Autodesk Inventor part; units mm, degrees
ref_plane "YZ Plane" through (0, 0, 0) normal (1, 0, 0) x (0, 1, 0)
ref_plane "XZ Plane" through (0, 0, 0) normal (0, 1, 0) x (-1, 0, 0)
ref_plane "XY Plane" through (0, 0, 0) normal (0, 0, 1) x (1, 0, 0)
sketch "Sketch1" plane through (0, 0, 0) normal (1, 0, 0) x (0, 1, 0)
  line L0 (35.589, 28.7672) -> (-47.596, 28.7672)
  line L1 (-47.596, 28.7672) -> (-47.596, 3.3672)
  line L2 (-47.596, 3.3672) -> (35.589, 3.3672)
  line L3 (35.589, 3.3672) -> (35.589, 28.7672)
  line L4 (-47.596, 20.8297) -> (-50.771, 20.8297)
  line L5 (-50.771, 20.8297) -> (-50.771, 11.3047)
  line L6 (-50.771, 11.3047) -> (-47.596, 11.3047)
  line L7 (-47.596, 11.3047) -> (-47.596, 20.8297)
  line L8 (-39.6585, 28.7672) -> (-30.1335, 28.7672)
  line L9 (-30.1335, 28.7672) -> (-30.1335, 25.5922)
  line L10 (-30.1335, 25.5922) -> (-39.6585, 25.5922)
  line L11 (-39.6585, 25.5922) -> (-39.6585, 28.7672)
  line L12 (-22.196, 20.8297) -> (-25.371, 20.8297)
  line L13 (-25.371, 20.8297) -> (-25.371, 11.3047)
  line L14 (-25.371, 11.3047) -> (-22.196, 11.3047)
  line L15 (-22.196, 11.3047) -> (-22.196, 20.8297)
  line L16 (-22.196, 3.3672) -> (-30.1335, 3.3672)
  line L17 (-30.1335, 3.3672) -> (-30.1335, 6.5422)
  line L18 (-30.1335, 6.5422) -> (-22.196, 6.5422)
  line L19 (-22.196, 6.5422) -> (-22.196, 3.3672)
  line L20 (-47.596, 3.3672) -> (-39.6585, 3.3672)
  line L21 (-39.6585, 3.3672) -> (-39.6585, 6.5422)
  line L22 (-39.6585, 6.5422) -> (-47.596, 6.5422)
  line L23 (-47.596, 6.5422) -> (-47.596, 3.3672)
  line L24 (35.589, 28.7672) -> (32.414, 28.7672)
  line L25 (32.414, 28.7672) -> (32.414, 20.8297)
  line L26 (32.414, 20.8297) -> (35.589, 20.8297)
  line L27 (35.589, 20.8297) -> (35.589, 28.7672)
  line L28 (35.589, 3.3672) -> (32.414, 3.3672)
  line L29 (32.414, 3.3672) -> (32.414, 11.3047)
  line L30 (32.414, 11.3047) -> (35.589, 11.3047)
  line L31 (35.589, 11.3047) -> (35.589, 3.3672)
  line L32 (27.6515, 3.3672) -> (18.1265, 3.3672)
  line L33 (18.1265, 3.3672) -> (18.1265, 6.5422)
  line L34 (18.1265, 6.5422) -> (27.6515, 6.5422)
  line L35 (27.6515, 6.5422) -> (27.6515, 3.3672)
  line L36 (27.6515, 28.7672) -> (18.1265, 28.7672)
  line L37 (18.1265, 28.7672) -> (18.1265, 25.5922)
  line L38 (18.1265, 25.5922) -> (27.6515, 25.5922)
  line L39 (27.6515, 25.5922) -> (27.6515, 28.7672)
  line L40 (13.364, 28.7672) -> (10.189, 28.7672)
  line L41 (10.189, 28.7672) -> (10.189, 20.8297)
  line L42 (10.189, 20.8297) -> (13.364, 20.8297)
  line L43 (13.364, 20.8297) -> (13.364, 28.7672)
  line L44 (13.364, 3.3672) -> (10.189, 3.3672)
  line L45 (10.189, 3.3672) -> (10.189, 11.3047)
  line L46 (10.189, 11.3047) -> (13.364, 11.3047)
  line L47 (13.364, 11.3047) -> (13.364, 3.3672)
  point P0 (0, 0)
  dimension "d0" = 25.4
  dimension "d1" = 3.175
  dimension "d2" = 7.9375
  dimension "d3" = 7.9375
  dimension "d4" = 83.185
  dimension "d5" = 3.175
  dimension "d6" = 9.525
  dimension "d7" = 7.9375
  dimension "d8" = 25.4
  dimension "d9" = 3.175
  dimension "d10" = 3.175
  dimension "d11" = 7.9375
  dimension "d12" = 3.175
  dimension "d13" = 7.9375
  dimension "d14" = 9.525
  dimension "d15" = 3.175
  dimension "d16" = 25.4
extrude "Extrusion1" add sketch "Sketch1" along normal blind 3.175 contours L25 L26 L3 L30 L29 L2 L35 L34 L33 L47 L46 L45 L19 L18 L17 L21 L22 L1 L0 L11 L10 L9 L41 L42 L43 L37 L38 L39 | L1 L6 L5 L4
For this review, take the finished solid that the model builds, in its own axes (mm). A direction names the side the tool comes from. Round coordinates to 2 decimals unless told otherwise and drop trailing zeros. Loops run counter-clockwise (first coordinate to the right, second up) from the corner with the lowest first, then second, coordinate; pieces in that order, holes last.
(1) Mouldability with a two-part tool opening along Y and no side actions: class faces 5 (the flat face through (2, -49, 20.83)), 6 (the flat face through (2, 27.652, 5)), 7 (the flat face through (2, -47.596, 25)) as released by +Y, released by -Y, zero draft, split by the parting line, or undercut.
Returned:
face 5: zero draft
face 6: undercut
face 7: released by -Y
(2) Tool access review of faces 1 (the flat face through (2, 18.126, 27)), 2 (the flat face through (2, -49, 11.305)), 3 (the flat face through (2, -26, 6.542)), 4 (the flat face through (2, -24, 20.83)): name each direction out of +Z, -Z, +X, -X, +Y, -Y from which nothing blocks a thin tool from reaching the whole face with its end or side.
Returned:
face 1: +Z, +X, -X
face 2: -Z, +X, -X, -Y
face 3: -Z, +X, -X
face 4: +X, -X
(3) We need section C-C (z = 10.25). Give the boundary of the cut face in (x, y) (3 decimals).
Returned:
outline: (0, -47.596) - (3.175, -47.596) - (3.175, 10.189) - (0, 10.189) - close; (0, 13.364) - (3.175, 13.364) - (3.175, 32.414) - (0, 32.414) - close
(4) Clearance check with flat-ended pins moving along their axes: P1, Ø1.6, axis at x = 2, z = 5, coming from the +Y side; P2, Ø1.6, axis at x = 1.5, y = 33.5, coming from the -Z side; P3, Ø1, axis at x = 1, z = 26.5, coming from the -Y side. State where each tip first meets the part, or that it passes through.
Returned:
P1: stops at y = 32.41
P2: stops at z = 11.3
P3: stops at y = -47.6
(5) We need section D-D (y = 23). Give the boundary of the cut face in (x, z) (3 decimals).
Returned:
outline: (0, 6.542) - (3.175, 6.542) - (3.175, 25.592) - (0, 25.592) - close
(6) We need section A-A (z = 27.25). Give the boundary of the cut face in (x, y) (1 decimal), plus the area to 3 significant figures.
Returned:
outline: (0, -47.6) - (3.2, -47.6) - (3.2, -39.7) - (0, -39.7) - close; (0, -30.1) - (3.2, -30.1) - (3.2, 10.2) - (0, 10.2) - close; (0, 13.4) - (3.2, 13.4) - (3.2, 18.1) - (0, 18.1) - close; (0, 27.7) - (3.2, 27.7) - (3.2, 32.4) - (0, 32.4) - close
area: 183 mm2
(7) We need section B-B (z = 17.75). Give the boundary of the cut face in (x, y) (3 decimals).
Returned:
outline: (0, -50.771) - (3.175, -50.771) - (3.175, -25.371) - (0, -25.371) - close; (0, -22.196) - (3.175, -22.196) - (3.175, 35.589) - (0, 35.589) - close
(8) Wall thickness on line 1 along Y through (x, z) = (1.15, 7.75); line 2 along Y through (x, z) = (2.9, 11.5); line 3 along Z through (x, y) = (1.55, 23): over which ranges is each line inside the solid? List them lowest first.
Returned:
line 1: y = -47.6 to 10.19, 13.36 to 32.41
line 2: y = -50.77 to -25.37, -22.2 to 35.59
line 3: z = 6.54 to 25.59
